Autodesk Inventor part; units mm, degrees
ref_plane "YZ Plane" through (0, 0, 0) normal (1, 0, 0) x (0, 1, 0)
ref_plane "XZ Plane" through (0, 0, 0) normal (0, 1, 0) x (-1, 0, 0)
ref_plane "XY Plane" through (0, 0, 0) normal (0, 0, 1) x (1, 0, 0)
sketch "スケッチ1" plane through (0, 0, 0) normal (0, 0, 1) x (1, 0, 0)
  line L0 (-2.75, 1.5877) -> (0, 3.1754)
  line L1 (0, 3.1754) -> (2.75, 1.5877)
  line L2 (2.75, 1.5877) -> (2.75, -1.5877)
  line L3 (2.75, -1.5877) -> (0, -3.1754)
  line L4 (0, -3.1754) -> (-2.75, -1.5877)
  line L5 (-2.75, -1.5877) -> (-2.75, 1.5877)
  circle A0 centre (0, 0) radius 1.5
  dimension "d0" = 5.5
  dimension "d1" = 3
extrude "押し出し1" add sketch "スケッチ1" along normal blind 12 contours L0 L1 L2 L3 L4 L5 | A0
sketch "スケッチ2" plane through (0, 0, 12) normal (0, 0, 1) x (1, 0, 0)
  circle A0 centre (0, 0) radius 1.5
  dimension "d4" = 3
extrude "押し出し2" add sketch "スケッチ2" along normal blind 6
extrude "押し出し3" add sketch "スケッチ1" against normal blind 6 contours A0
properties part number "スペーサー　両雄ねじ　m3-12" material "アルミニウム 2014-T4"
Build history of the part. All positions in model axes, mm. A direction names the side the tool comes from. Coordinates: 2 decimals unless noted, no trailing zeros. Order: outer loops, then holes, each group sorted by start corner. A loop starts at its lowest first (then second) coordinate and runs counter-clockwise, first axis right, second up. Notation, with made-up numbers: M 55.25,82 L 113.25,82 A27 ccw 113.25,113 Z; hole C 17,-2.75 d6. An arc over 180 degrees is marked long. One line per question, with ' | ' between items. Start each with the question number.
1. Cut at B-B (z = 3). Write the cut outline in (x, y), plus the area to 3 significant figures.
2. Cut at A-A (y = 0). Write the cut outline in (x, z).
3. Tool access for faces 1 (the face through (-1.5, 0.07, -2.96)), 2 (the face through (-1.5, -0.07, 14.96)), 3 (the face through (-1.36, -2.39, 5.92)): list every direction of +Z, -Z, +X, -X, +Y, -Y with a clear straight run to the whole face (end or side of a thin tool).
4. Flat gauge pins, fed straight in: P1, Ø3, axis at y = 0, z = -3, coming from the +X side; P2, Ø2, axis at x = 0.5, y = 2, coming from the +Z side. Where does each tip first touch, or does it go through?
5. Cut at C-C (x = -1.2). Write the cut outline in (y, z), plus the area to 3 significant figures.
6. Wall check: line 1 along Y through (x, z) = (-0.1, -1.25); line 2 along Z through (x, y) = (1, 2.5); line 3 along Y through (x, z) = (-1.75, 8.5). Give the ranges that are in metal, low to high. Write a range as [from, to].
7. Cut at D-D (z = 16.5). Write the cut outline in (x, y).
The answers:
1) outline: M -2.75,-1.59 L 0,-3.18 L 2.75,-1.59 L 2.75,1.59 L 0,3.18 L -2.75,1.59 Z | area: 26.2 mm2
2) outline: M -2.75,0 L -1.5,0 L -1.5,-6 L 1.5,-6 L 1.5,0 L 2.75,0 L 2.75,12 L 1.5,12 L 1.5,18 L -1.5,18 L -1.5,12 L -2.75,12 Z
3) face 1: -Z | face 2: +Z | face 3: +Z, -Z, -X, -Y
4) P1: stops at x = 1.5 | P2: stops at z = 18
5) outline: M -2.48,0 L -0.9,0 L -0.9,-6 L 0.9,-6 L 0.9,0 L 2.48,0 L 2.48,12 L 0.9,12 L 0.9,18 L -0.9,18 L -0.9,12 L -2.48,12 Z | area: 81.2 mm2
6) line 1: y = [-1.5, 1.5] | line 2: z = [0, 12] | line 3: y = [-2.17, 2.17]
7) outline: C 0,0 d3
